Read the model definition and answer for the solid it produces. Units are mm, in the model's axes. A direction names the side the tool comes from. Coordinates: 2 decimals unless noted, no trailing zeros. Loops run counter-clockwise (first coordinate to the right, second up) from the corner with the lowest first, then second, coordinate; pieces in that order, holes last. Notation, with made-up numbers: (58.5, -9) -> (78.5, -9) arc R24 cw to (78.5, 3) -> close; hole circle Ø2 at (40.25, 79.25). An arc over 180 degrees is marked (long way). One line per question, with ' | ' between items. Start each with the question number.
```python
from build123d import *

# Parameters (mm, degrees)
F0_W     = 19.05
F0_H     = 0.635
F2_DEPTH = 12.7
F3_R     = 11.037784


with BuildPart() as f1:
    # F0 (on Front) → F1 (revolve)
    with BuildSketch(Plane.XZ):
        Polygon((0, 0), (0, 6.35), (-50.8, 6.35), (-50.8, 0.635), (-50.8, 0), align=None)
        Polygon((76.2, 12.7), (0, 12.7), (0, 6.35), (0, 0), (76.2, 0), align=None)
        Polygon((-50.8, 0.635), (-50.8, 6.35), (-69.85, 0.635), align=None)
        with Locations((-60.325, 0.3175)):
            Rectangle(F0_W, F0_H)
        Polygon((-69.85, 0.635), (-50.8, 6.35), (-69.85, 6.35), align=None)
    revolve(axis=Axis((3.175, 0, 0), (-1, 0, 0)))

    # F0 (on Front) → F2 (cut, symmetric)
    with BuildSketch(Plane.XZ):
        Polygon((-69.85, 0.635), (-50.8, 6.35), (-69.85, 6.35), align=None)
        Polygon((-69.85, -6.35), (-50.8, -6.35), (-69.85, -0.635), align=None)
    extrude(amount=F2_DEPTH, both=True, mode=Mode.SUBTRACT)

    # F3
    f3_edges = [f1.edges().sort_by_distance(p)[0] for p in [
        (76.2, 0, -12.7),
    ]]
    fillet(f3_edges, radius=F3_R)


solid = f1.part
```
(1) Section B-B on x = -52.5 is taken. Write down the section's boundary in (y, z), plus the area to 3 significant figures.
(2) Find the intervals of material crossed by probe 1 along Y at (x, z) = (41.5, 0); probe 2 along Z at (x, y) = (36, -10.75); probe 3 along Z at (x, y) = (3, 10), in increasing order. Write a range as from..to.
(3) Each of these flat-tipped pins is pushed along its axis until it touches: pin 1 Ø12 at (y, z) = (1.5, 10) entering from +X; pin 2 Ø1.5 at (x, z) = (-54.5, 5.5) entering from +Y; pin 3 Ø10 at (x, y) = (-53.5, 0.5) entering from -Z. Where does it stop, or does it pass through?
(4) A tool of negligible diameter and unlimited length cuts with its end or side. For faces 1 (the flat face through (0, 6, 3)), 2 (the cylindrical face through (32.12, -12.4, -2.75)), from which of +Z, -Z, +X, -X, +Y, -Y can it reach the whole face along a straight path? Write none if from no direction.
(5) Section A-A on x = 43.5 is taken. Write down the section's boundary in (y, z).
Working result:
1) outline: (-2.49, -5.84) -> (2.49, -5.84) arc R6.35 ccw to (2.49, 5.84) -> (-2.49, 5.84) arc R6.35 ccw to start | area: 123 mm2
2) probe 1: y = -12.7..12.7 | probe 2: z = -6.76..6.76 | probe 3: z = -7.83..7.83
3) pin 1: stops at x = 75.92 | pin 2: stops at y = 4.21 | pin 3: stops at z = -6.35
4) face 1: -X | face 2: +X, -X
5) outline: circle Ø25.4 at (0, 0)
